Part print with two shaded views. Sizes in mm from the minimum x, y, z corner. A direction names the side the tool comes from. Give positions to 0.01 mm unless a question says otherwise; leave off trailing zeros. Write each loop counter-clockwise with the first axis right and the second up, starting at its lowest first coordinate (ties: lowest second). Pieces come first, ordered by that corner, then holes. Notation, with made-up numbers: (70.25, 76) -> (127.25, 76) arc R31 cw to (127.25, 114) -> close; hole circle Ø9 at (-32, 86). An arc over 180 degrees is marked (long way). Answer as a JSON object with one key per item and string values.
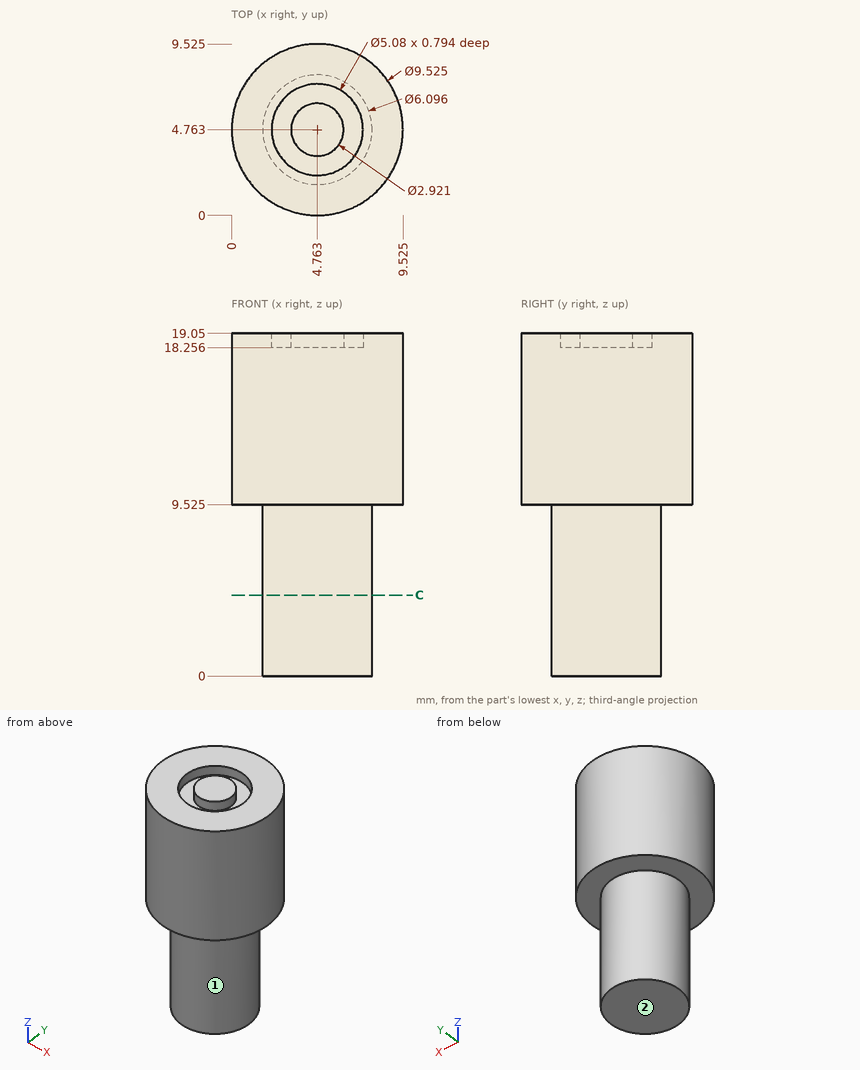
1) Wall check: probe 1 along Z at (x, y) = (6.25, 6.25); probe 2 along Y at (x, z) = (1.25, 15) (1 decimal); probe 3 along Y at (x, z) = (5, 17.5) (1 decimal). Give the ranges that are in metal, low to high.
Model answer:
{"probe 1": "z = 0 to 18.26", "probe 2": "y = 1.5 to 8", "probe 3": "y = 0 to 9.5"}
2) 3-axis set-ups, long thin cutter, end or side, ignore diameter. For the marked faces 1 and 2: which of +Z, -Z, +X, -X, +Y, -Y reach the whole face in a straight line?
Model answer:
{"face 1": "-Z", "face 2": "-Z, +X, -X, +Y, -Y"}
3) Slice it at C-C (z = 4.5). List the corners of the cut face in (x, y) (1 decimal), then the cut area to 3 significant figures.
Model answer:
{"outline": "circle Ø6.1 at (4.8, 4.8)", "area": "29.2 mm2"}
4) Pin check, flat tip, straight feed: pin 1 (3 mm diameter, centred on x = 1.5, z = 5.5, fed in from -Y) (1 decimal). Stop position of the tip, or through.
Model answer:
{"pin 1": "stops at y = 2.3"}
